```python
from build123d import *

# Parameters (mm, degrees)
SKETCH1_W           = 76.2
SKETCH1_H           = 139.7
BOSS_EXTRUDE1_DEPTH = 25.4
FILLET1_R           = 2.54
SHELL1_START        = -110.973034188
SHELL1_OUTLINE_W    = 20.32
SHELL1_OUTLINE_H    = 134.62
SHELL1_DEPTH        = 71.12
SKETCH5_W           = 71.12
SKETCH5_H           = 134.62
CUT_EXTRUDE1_DEPTH  = 25.4


# Read off the part's stored shape, not the designer's step: Shell1
with BuildPart() as part:
    # Sketch1 → Boss-Extrude1 (new body)
    with BuildSketch(Plane(origin=(0, 0, 0), x_dir=(1, 0, 0), z_dir=(0, 1, 0))):
        with Locations((-75.413034188, -14.477457265)):
            Rectangle(SKETCH1_W, SKETCH1_H)
    extrude(amount=BOSS_EXTRUDE1_DEPTH)

    # Fillet1
    fillet1_edges = [part.edges().sort_by_distance(p)[0] for p in [
        (-75.413034188, 0, -55.372542735),
        (-37.313034188, 0, 14.477457265),
        (-75.413034188, 0, 84.327457265),
        (-113.513034188, 0, 14.477457265),
        (-113.513034188, 12.7, -55.372542735),
        (-37.313034188, 12.7, -55.372542735),
        (-37.313034188, 12.7, 84.327457265),
        (-113.513034188, 12.7, 84.327457265),
    ]]
    fillet(fillet1_edges, radius=FILLET1_R)

    # Shell1 outline → Shell1 (cut)
    with BuildSketch(Plane.YZ.offset(SHELL1_START)):
        with Locations((12.7, 14.477457265)):
            Rectangle(SHELL1_OUTLINE_W, SHELL1_OUTLINE_H)
    extrude(amount=SHELL1_DEPTH, mode=Mode.SUBTRACT)

    # Sketch5 → Cut-Extrude1 (cut)
    with BuildSketch(Plane(origin=(0, 25.4, 0), x_dir=(1, 0, 0), z_dir=(0, 1, 0))):
        with Locations((-75.413034188, -14.477457265)):
            Rectangle(SKETCH5_W, SKETCH5_H)
    extrude(amount=-CUT_EXTRUDE1_DEPTH, mode=Mode.SUBTRACT)


solid = part.part
```
Part model, mm, in its own coordinate system. A direction names the side the tool comes from. Round coordinates to 2 decimals unless told otherwise and drop trailing zeros. Loops run counter-clockwise (first coordinate to the right, second up) from the corner with the lowest first, then second, coordinate; pieces in that order, holes last.
Item 1: Cut at B-B, the plane z = -26. Give the cut face in (x, y), then the cut area to 3 significant figures.
Item 2: Cut at C-C, the plane y = 4.25. Give the cut face in (x, z), then the cut area to 3 significant figures.
Item 3: Mould opens along Z. For faces 3 (the face through (-39.853, 13, 15)), 4 (the face through (-112.79, 14.13, 83.56)), 5 (the face through (-38.04, 14.13, -54.61)) say: +Z half, -Z half, draft (parallel to the pull), parting line (faces both ways), or undercut.
Item 4: 3-axis set-ups, long thin cutter, end or side, ignore diameter. For faces 1 (the face through (-112.789, 0.764, 13.535)), 2 (the face through (-110.973, 13, 15)): which of +Z, -Z, +X, -X, +Y, -Y reach the whole face in a straight line?
Item 5: Drill centre lines: line 1 (X direction, y = 17, z = 36.5); line 2 (Z direction, x = -97.5, y = 10.5); line 3 (X direction, y = 1.25, z = 39.5) (3 decimals). Where is each one in solid material? Low to high.
Item 6: Cut at A-A, the plane x = -90. Give the cut face in (y, z).
A:
1. outline: (-113.51, 2.54) arc R2.54 ccw to (-110.97, 0) - (-110.97, 25.4) - (-113.51, 25.4) - close; (-39.85, 0) arc R2.54 ccw to (-37.31, 2.54) - (-37.31, 25.4) - (-39.85, 25.4) - close
1. area: 126 mm2
2. outline: (-113.51, -52.83) arc R2.54 ccw to (-110.97, -55.37) - (-39.85, -55.37) arc R2.54 ccw to (-37.31, -52.83) - (-37.31, 81.79) arc R2.54 ccw to (-39.85, 84.33) - (-110.97, 84.33) arc R2.54 ccw to (-113.51, 81.79) - close; hole (-110.97, -52.83) - (-39.85, -52.83) - (-39.85, 81.79) - (-110.97, 81.79) - close
2. area: 1,070 mm2
3. face 3: undercut
3. face 4: +Z half
3. face 5: -Z half
4. face 1: +Z, -Z, -X, -Y
4. face 2: +Y, -Y
5. line 1: x = -113.51 to -110.97, -39.85 to -37.31
5. line 2: z = -55.37 to -52.83, 81.79 to 84.33
5. line 3: x = -113.161 to -110.973, -39.853 to -37.665
6. outline: (0, -52.83) arc R2.54 ccw to (2.54, -55.37) - (25.4, -55.37) - (25.4, -52.83) - close; (0, 81.79) - (25.4, 81.79) - (25.4, 84.33) - (2.54, 84.33) arc R2.54 ccw to start
